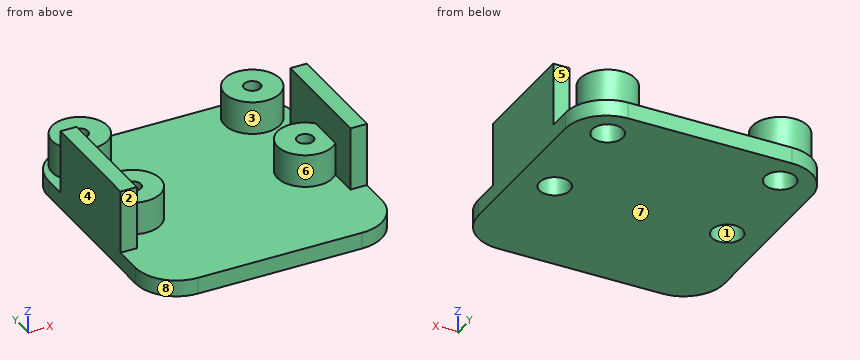
```python
from build123d import *

# Parameters (mm, degrees)
F0_W     = 30
F0_H     = 30.25
F1_DEPTH = 2
F2_W     = 2
F2_H     = 14
F3_DEPTH = 7.75
F5_R     = 3.375
F6_DEPTH = 6
F4_R     = 1.875
F7_DEPTH = 4
F9_D     = 2
F9_DEPTH = 4
F9_START = 4
F9_TIP   = 0.600860619
F10_R    = 5


with BuildPart() as f1:
    # F0 (on Top) → F1 (new body)
    with BuildSketch(Plane.XY):
        Rectangle(F0_W, F0_H)
    extrude(amount=F1_DEPTH)

    # F2 (on face) → F3 (join)
    with BuildSketch(Plane.XY.offset(2)):
        with Locations((-14, 0.325)):
            Rectangle(F2_W, F2_H)
        with Locations((14, 0.325)):
            Rectangle(F2_W, F2_H)
    extrude(amount=F3_DEPTH)

    # F5 (on face) → F6 (join)
    with BuildSketch(Plane(origin=(0, 0, 0), x_dir=(1, 0, 0), z_dir=(0, 0, -1))):
        with Locations((10.5, -11.375)):
            Circle(F5_R)
        with Locations((-10.5, -11.375)):
            Circle(F5_R)
        with Locations((-10.5, 0.925)):
            Circle(F5_R)
        with Locations((10.5, 0.925)):
            Circle(F5_R)
    extrude(amount=-F6_DEPTH)

    # F4 (on face) → F7 (cut)
    with BuildSketch(Plane(origin=(0, 0, 0), x_dir=(1, 0, 0), z_dir=(0, 0, -1))):
        with Locations((-10.5, -11.375)):
            Circle(F4_R)
        with Locations((-10.5, 0.925)):
            Circle(F4_R)
        with Locations((10.5, -11.375)):
            Circle(F4_R)
        with Locations((10.5, 0.925)):
            Circle(F4_R)
    extrude(amount=-F7_DEPTH, mode=Mode.SUBTRACT)

    # F9
    # its depths count from where the whole tool has entered the part; down to there all is cleared
    with Locations(Plane(origin=(0, 0, 0), x_dir=(1, 0, 0), z_dir=(0, 0, -1)).offset(-F9_START)):
        with Locations((-10.5, 0.925), (-10.5, -11.375), (10.5, -11.375), (10.5, 0.925)):
            Hole(F9_D / 2, depth=F9_DEPTH)
            with Locations((0, 0, -(F9_DEPTH + F9_TIP / 2))):  # 118° drill point
                Cone(0, F9_D / 2, F9_TIP, mode=Mode.SUBTRACT)

    # F10
    f10_edges = [f1.edges().sort_by_distance(p)[0] for p in [
        (-15, -15.125, 1),
        (15, -15.125, 1),
        (15, 15.125, 1),
        (-15, 15.125, 1),
    ]]
    fillet(f10_edges, radius=F10_R)


solid = f1.part
```
The model under review builds one solid part; all positions refer to its coordinate system, in mm. Face numbers are marked on the shaded views. A direction names the side the tool comes from. Round coordinates to 2 decimals unless told otherwise and drop trailing zeros. Loops run counter-clockwise (first coordinate to the right, second up) from the corner with the lowest first, then second, coordinate; pieces in that order, holes last. Notation, with made-up numbers: M 89.5,67 L 134.5,67 A10 cw 134.5,81 Z; hole C -0.5,0.25 d5. An arc over 180 degrees is marked long. Write item = value, one per line.
Item 1: The part is to be moulded in two halves that separate along X. For the marked faces 6, 7 and 8, say which applies: released by +X, released by -X, zero draft, split by the parting line, or undercut.
Return value:
face_6 = undercut
face_7 = zero draft
face_8 = released by -X
Item 2: Take a section at C-C on z = 4.5. Write out the cut boundary in (x, y) (3 decimals), then the cut area to 3 significant figures.
Return value:
outline = M -15,-6.675 L -13,-6.675 L -13,-3.192 A3.375 ccw long -13,1.342 L -13,7.325 L -15,7.325 Z; C -10.5,11.375 d6.75; C 10.5,11.375 d6.75; M 13,-6.675 L 15,-6.675 L 15,7.325 L 13,7.325 L 13,1.342 A3.375 ccw long 13,-3.192 Z; hole C -10.5,-0.925 d2; hole C -10.5,11.375 d2; hole C 10.5,-0.925 d2; hole C 10.5,11.375 d2
area = 181 mm2
Item 3: Take a section at D-D on y = 12. Write out the cut boundary in (x, z), then the cut area to 3 significant figures.
Return value:
outline = M -14.64,0 L -12.27,0 L -12.27,4 L -11.28,4 L -11.28,6 L -13.82,6 L -13.82,2 L -14.64,2 Z; M -9.72,4 L -8.73,4 L -8.73,0 L 8.73,0 L 8.73,4 L 9.72,4 L 9.72,6 L 7.18,6 L 7.18,2 L -7.18,2 L -7.18,6 L -9.72,6 Z; M 11.28,4 L 12.27,4 L 12.27,0 L 14.64,0 L 14.64,2 L 13.82,2 L 13.82,6 L 11.28,6 Z
area = 77.1 mm2
Item 4: For line 1 (Y direction, x = -10.5, z = 5.35) (3 decimals); line 2 (Y direction, x = 10.5, z = 2.45); line 3 (X direction, y = 5.5, z = 6.75), list the stretches that pass through material, from the lowest coordinate up. Write a range as [from, to].
Return value:
line_1 = [-4.3, -1.925], [0.075, 2.45], [8, 10.375], [12.375, 14.75]
line_2 = [-4.3, -2.8], [0.95, 2.45], [8, 9.5], [13.25, 14.75]
line_3 = [-15, -13], [13, 15]
Item 5: Machinability: for the marked faces 1, 2, 3, 4 and 5, which of the approach directions +Z, -Z, +X, -X, +Y, -Y give a long, thin tool a straight path to every point of the face, cutting with its end or side? Answer none if there is none.
Return value:
face_1 = -Z
face_2 = +Z, +X, -X, -Y
face_3 = +Z
face_4 = +Z, -Z, -X, +Y, -Y
face_5 = +Z, +X, -X
Item 6: Take a section at A-A on z = 8. Write out the cut boundary in (x, y) (3 decimals), then the cut area to 3 significant figures.
Return value:
outline = M -15,-6.675 L -13,-6.675 L -13,7.325 L -15,7.325 Z; M 13,-6.675 L 15,-6.675 L 15,7.325 L 13,7.325 Z
area = 56.0 mm2
Item 7: Insertion check: P1, Ø1.9, axis at x = -11, y = 11, coming from the -Z side; P2, Ø1.8, axis at x = 10.5, y = -0.925, coming from the +Z side; P3, Ø5.5, axis at x = -10, y = 10.5, coming from the +Z side; P4, Ø1.6, axis at x = 13.5, z = 7, coming from the +Y side (3 decimals). Each pin has a flat end and moves straight along its axis. Give the tip position at first contact, or say it passes through.
Return value:
P1 = 4
P2 = through
P3 = 6
P4 = 7.325
Item 8: Take a section at B-B on x = -11. Write out the cut boundary in (y, z), then the cut area to 3 significant figures.
Return value:
outline = M -15.02,0 L -2.73,0 L -2.73,4 L -1.79,4 L -1.79,6 L -4.26,6 L -4.26,2 L -15.02,2 Z; M -0.06,4 L 0.88,4 L 0.88,0 L 9.57,0 L 9.57,4 L 10.51,4 L 10.51,6 L 8.04,6 L 8.04,2 L 2.41,2 L 2.41,6 L -0.06,6 Z; M 12.24,4 L 13.18,4 L 13.18,0 L 15.02,0 L 15.02,2 L 14.71,2 L 14.71,6 L 12.24,6 Z
area = 77.7 mm2
